Read the model definition and answer for the solid it produces. Units are mm, in the model's axes. A direction names the side the tool comes from. Round coordinates to 2 decimals unless told otherwise and drop trailing zeros. Order: outer loops, then holes, each group sorted by start corner. A loop starts at its lowest first (then second) coordinate and runs counter-clockwise, first axis right, second up. Notation, with made-up numbers: (-7.75, 12.5) -> (-0.75, 12.5) arc R16 cw to (-0.75, 42.5) -> close; hole circle Ø7 at (15, 54.5). An arc over 180 degrees is marked (long way). Answer as a JSON object with one key per item and string values. Group by question number.
Item 1: Section C-C, the plane y = 2.65 is taken. Write down the section's boundary in (x, z), plus the area to 3 significant figures.
Item 2: Section A-A, the plane z = -20 is taken. Write down the section's boundary in (x, y).
Item 3: For faces 1 (the flat face through (-27.75, 2, 0)), 2 (the flat face through (-5, 0, 0)), determine the directions among +Z, -Z, +X, -X, +Y, -Y from which every point of the face is accessible in a straight line to the end or side of a thin tool.
Item 4: Section B-B, the plane x = -3 is taken. Write down the section's boundary in (y, z).
Item 5: Consider probe 1 along Y at (x, z) = (-25, 2.5); probe 2 along X at (y, z) = (2.1, 20); probe 3 along Y at (x, z) = (27, -3.5). Determine where each line is inside the solid, lowest interval first. Write a range as from..to.
Item 6: Given P1, Ø6, axis at x = -23.5, z = -8.5, coming from the +Y side; P2, Ø0.9, axis at y = 2.5, z = -8, coming from the +X side, each flat-ended and moving along its own axis, determine where each tip first touches the part or whether it passes through.
from build123d import *

# Parameters (mm, degrees)
SKETCH1_W           = 60
SKETCH1_H           = 60
BOSS_EXTRUDE1_DEPTH = 1.5
SKETCH4_W           = 2.25
SKETCH4_H           = 60
BOSS_EXTRUDE2_DEPTH = 1.85
CHAMFER1_SIZE       = 10
CHAMFER1_SIZE2      = 0.874886635


with BuildPart() as part:
    # Sketch1 → Boss-Extrude1 (new body)
    with BuildSketch(Plane(origin=(0, 0, 0), x_dir=(1, 0, 0), z_dir=(0, 1, 0))):
        Rectangle(SKETCH1_W, SKETCH1_H)
    extrude(amount=BOSS_EXTRUDE1_DEPTH)

    # Sketch4 → Boss-Extrude2 (add)
    with BuildSketch(Plane(origin=(0, 1.5, 0), x_dir=(1, 0, 0), z_dir=(0, 1, 0))):
        with Locations((-28.875, 0)):
            Rectangle(SKETCH4_W, SKETCH4_H)
    extrude(amount=BOSS_EXTRUDE2_DEPTH)

    # Chamfer1
    chamfer1_edges = [part.edges().sort_by_distance(p)[0] for p in [
        (30, 0, 0),
    ]]
    chamfer1_side = [part.faces().sort_by_distance(p)[0] for p in [
        (0, 0, 0),
    ]]
    chamfer(chamfer1_edges, length=CHAMFER1_SIZE, length2=CHAMFER1_SIZE2, reference=chamfer1_side[0])


solid = part.part
Values found:
{
 "1": {"outline": "(-30, -30) -> (-27.75, -30) -> (-27.75, 30) -> (-30, 30) -> close", "area": "135 mm2"},
 "2": {"outline": "(-30, 0) -> (20, 0) -> (30, 0.87) -> (30, 1.5) -> (-27.75, 1.5) -> (-27.75, 3.35) -> (-30, 3.35) -> close"},
 "3": {"face 1": "+Z, -Z, +X, +Y", "face 2": "+Z, -Z, +X, -X, -Y"},
 "4": {"outline": "(0, -30) -> (1.5, -30) -> (1.5, 30) -> (0, 30) -> close"},
 "5": {"probe 1": "0..1.5", "probe 2": "-30..-27.75", "probe 3": "0.61..1.5"},
 "6": {"P1": "y = 1.5", "P2": "x = -27.75"}
}
